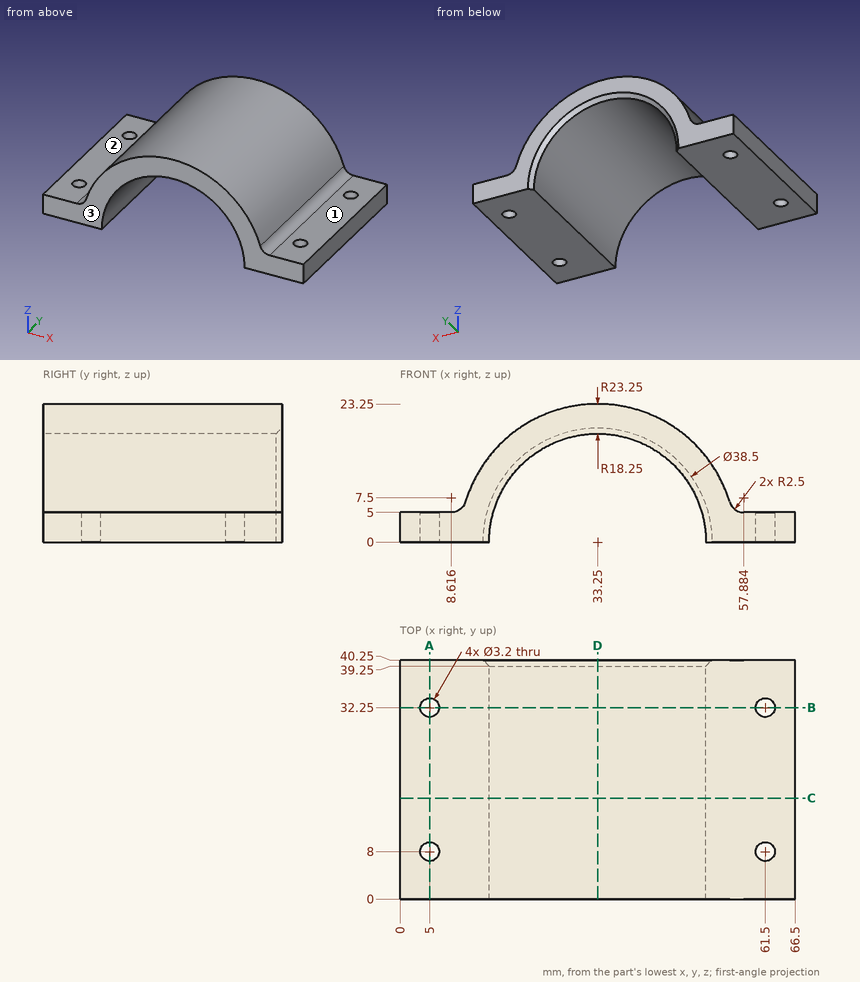
Answer from the drawing. Dimensions are ordinates in mm from the lowest x, y and z of the part. A direction names the side the tool comes from. Round coordinates to 2 decimals unless told otherwise and drop trailing zeros. Loops run counter-clockwise (first coordinate to the right, second up) from the corner with the lowest first, then second, coordinate; pieces in that order, holes last.
(1) The part is cut by section B-B, the plane y = 32.25. Give the vertices of the cut face in (x, z), and give its area (3 significant figures).
Computed values:
outline: (0, 0) - (3.4, 0) - (3.4, 5) - (0, 5) - close; (6.6, 0) - (15, 0) arc R18.25 cw to (51.5, 0) - (59.9, 0) - (59.9, 5) - (57.88, 5) arc R2.5 cw to (55.49, 6.77) arc R23.25 ccw to (11.01, 6.77) arc R2.5 cw to (8.62, 5) - (6.6, 5) - close; (63.1, 0) - (66.5, 0) - (66.5, 5) - (63.1, 5) - close
area: 397 mm2
(2) The part is cut by section C-C, the plane y = 17. Give the vertices of the cut face in (x, z).
Computed values:
outline: (0, 0) - (15, 0) arc R18.25 cw to (51.5, 0) - (66.5, 0) - (66.5, 5) - (57.88, 5) arc R2.5 cw to (55.49, 6.77) arc R23.25 ccw to (11.01, 6.77) arc R2.5 cw to (8.62, 5) - (0, 5) - close
(3) The part is cut by section D-D, the plane x = 33.25. Give the vertices of the cut face in (y, z).
Computed values:
outline: (0, 18.25) - (39.25, 18.25) - (40.25, 19.25) - (40.25, 23.25) - (0, 23.25) - close
(4) For the marked faces 1, 2 and 3, determine the directions among +Z, -Z, +X, -X, +Y, -Y from which every point of the face is accessible in a straight line to the end or side of a thin tool.
Computed values:
face 1: +Z, +X, +Y, -Y
face 2: +Z, -X, +Y, -Y
face 3: +Z, -Z, +X, -X, -Y
(5) Each of these flat-tipped pins is pushed along its axis until it touches: P1, Ø1, axis at x = 9.5, y = 20, coming from the +Z side; P2, Ø4, axis at x = 5, y = 8, coming from the +Z side; P3, Ø3, axis at x = 43.5, y = 29.5, coming from the -Z side (1 decimal). Where does it stop, or does it pass through?
Computed values:
P1: stops at z = 5.42
P2: stops at z = 5
P3: stops at z = 14
(6) Find the intervals of material crossed by L1, parallel to Y at x = 5, z = 1.2; L2, parallel to Z at x = 60.5, y = 16; L3, parallel to X at y = 9, z = 6.5, in increasing order.
Computed values:
L1: y = 0 to 6.4, 9.6 to 30.65, 33.85 to 40.25
L2: z = 0 to 5
L3: x = 10.91 to 16.2, 50.3 to 55.59
(7) The part is cut by section A-A, the plane x = 5. Give the vertices of the cut face in (y, z), and give its area (3 significant figures).
Computed values:
outline: (0, 0) - (6.4, 0) - (6.4, 5) - (0, 5) - close; (9.6, 0) - (30.65, 0) - (30.65, 5) - (9.6, 5) - close; (33.85, 0) - (40.25, 0) - (40.25, 5) - (33.85, 5) - close
area: 169 mm2
